Can you work these out from the model? Positions are in its coordinate system, mm. Face numbers are marked on the shaded views. A direction names the side the tool comes from. Give positions to 0.01 mm unless a question says otherwise; leave off trailing zeros. Write each loop counter-clockwise with the first axis right and the second up, starting at its lowest first coordinate (ties: lowest second). Pieces come first, ordered by that corner, then holes.
1. Suppose I cut it at D-D (z = -1.5). Please give me the cut outline in (x, y), and give its area (3 significant figures).
2. If I drill on probe 1 along Z at (x, y) = (3.4, 0); probe 2 along Z at (x, y) = (3.2, 0); probe 3 along Y at (x, z) = (3.8, 0.75), over which ranges is the centre line in solid material (lowest first)?
3. I'm going to push flat-ended pins straight in: pin 1 (2 mm diameter, centred on y = 0, z = 2.5, fed in from -X); pin 2 (1.5 mm diameter, centred on x = 2.5, z = 1, fed in from +Y); pin 3 (2 mm diameter, centred on x = 3, y = 1, fed in from +Z). Where does each tip first touch, or does it pass through?
4. On a 3-axis mill with a long thin cutter (end or side, diameter ignored), from which of +Z, -Z, +X, -X, +Y, -Y can I reach the whole of each face in a straight line? I mean the marked faces 1 and 2. Say none if no direction works.
5. Thinking about a two-plate mould opening in Y: for the marked faces 3, 4 and 5, which applies, pulls with the +Y half, pulls with the -Y half, needs draft (parallel to the pull), parting line crosses it, or undercut?
6. Suppose I cut it at C-C (x = 3). Please give me the cut outline in (y, z).
7. Suppose I cut it at B-B (x = 1.8). Please give me the cut outline in (y, z).
8. Suppose I cut it at A-A (z = 0.75). Please give me the cut outline in (x, y), and give its area (3 significant figures).
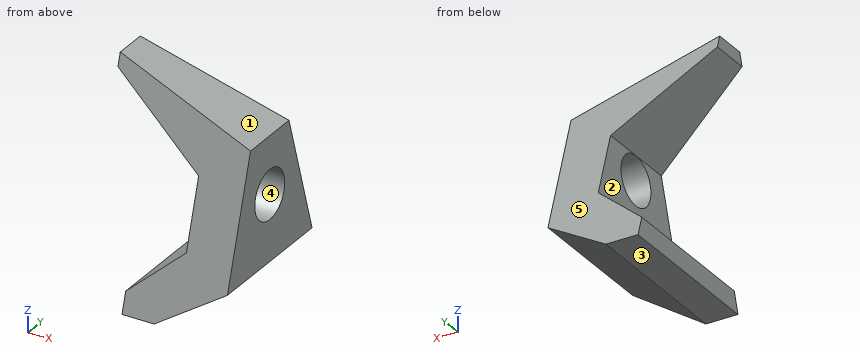
```python
from build123d import *

# Parameters (mm, degrees)
F1_DEPTH = 4.25
F2_R     = 0.75
F3_DEPTH = 4.251
F5_DEPTH = 12.7


with BuildPart() as f1:
    # F0 (on Right) → F1 (new body)
    with BuildSketch(Plane.YZ):
        Polygon((0.5, 4), (-0.5, 4), (-2.5, -2.5), (2.5, -2.5), align=None)
    extrude(amount=F1_DEPTH)

    # F2 (on face) → F3 (cut, through all)
    with BuildSketch(Plane.YZ.offset(4.25)):
        with Locations((0, 0.75)):
            Circle(F2_R)
    extrude(amount=-F3_DEPTH, mode=Mode.SUBTRACT)

    # F4 (on Front) → F5 (cut, symmetric)
    with BuildSketch(Plane.XZ):
        Polygon((2.8575, 1.5), (0, 3.619), (0, -2.5), (1.27, -2.5), (1.27, -1.8904), (2.8575, -0.5), align=None)
        Polygon((4.25, 2.5), (4.25, 4), (0, 4), align=None)
        Polygon((2.25, -2.5), (4.25, -2.5), (4.25, -1.25), align=None)
    extrude(amount=F5_DEPTH, both=True, mode=Mode.SUBTRACT)


solid = f1.part
```
Checks:
1. outline: (1.72, -2.19) - (3.85, -2.19) - (3.85, 2.19) - (1.72, 2.19) - close
1. area: 9.36 mm2
2. probe 1: z = -1.78 to 0, 1.5 to 2.8
2. probe 2: z = -1.91 to 0, 1.5 to 2.87
2. probe 3: y = -1.5 to -0.75, 0.75 to 1.5
3. pin 1: stops at x = 0.16
3. pin 2: stops at y = 1.63
3. pin 3: stops at z = 3.28
4. face 1: +Z, +X, +Y, -Y
4. face 2: -X, +Y, -Y
5. face 3: needs draft
5. face 4: undercut
5. face 5: pulls with the +Y half
6. outline: (-2.36, -2.03) - (2.36, -2.03) - (0.83, 2.94) - (-0.83, 2.94) - close; hole circle Ø1.5 at (0, 0.75)
7. outline: (-2.5, -2.5) - (2.5, -2.5) - (2.17, -1.43) - (-2.17, -1.43) - close; (-1.03, 2.28) - (1.03, 2.28) - (0.7, 3.36) - (-0.7, 3.36) - close
8. outline: (2.86, -1.5) - (4.25, -1.5) - (4.25, -0.75) - (2.86, -0.75) - close; (2.86, 0.75) - (4.25, 0.75) - (4.25, 1.5) - (2.86, 1.5) - close
8. area: 2.09 mm2
